Design review of the part built by this model. Coordinates are the model's own, in mm. Face numbers are marked on the shaded views. A direction names the side the tool comes from. Round coordinates to 2 decimals unless told otherwise and drop trailing zeros. Loops run counter-clockwise (first coordinate to the right, second up) from the corner with the lowest first, then second, coordinate; pieces in that order, holes last. Notation, with made-up numbers: M -14.75,82 L 41.25,82 A31 ccw 41.25,108 Z; hole C -39,8 d6. An arc over 180 degrees is marked long. Answer as CSV lines item,"result". Start each with the question number.
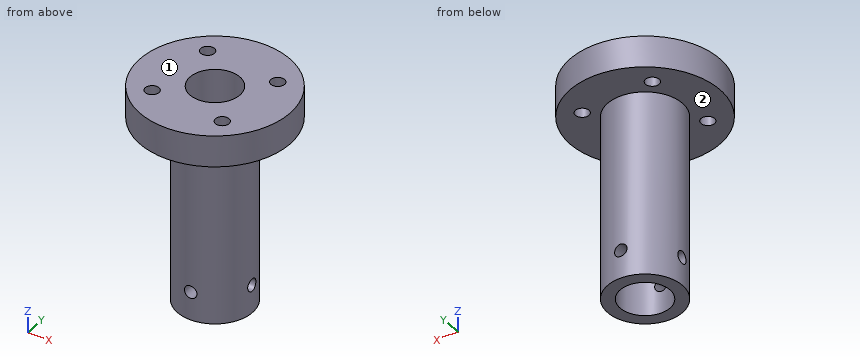
from build123d import *

# Parameters (mm, degrees)
SKIZZE1_R                            = 12.5
AUFSATZ_LINEAR_AUSTRAGEN1_DEPTH      = 40
SCHNITT_LINEAR_START                 = 30
SKIZZE4_R                            = 15
SKIZZE4_R_2                          = 12
SCHNITT_LINEAR_AUSTRAGEN1_DEPTH      = 20
SKIZZE5_R                            = 1.1
SCHNITT_LINEAR_AUSTRAGEN2_DEPTH      = 20
SKIZZE6_R                            = 1
SCHNITT_LINEAR_AUSTRAGEN3_DEPTH      = 10
SKIZZE8_W                            = 5.5
SKIZZE8_H                            = 25
SCHNITT_LINEAR_AUSTRAGEN5_DEPTH      = 13.5
SCHNITT_LINEAR_AUSTRAGEN5_DEPTH_BACK = 13.5
SKIZZE9_R                            = 1
SCHNITT_LINEAR_AUSTRAGEN6_DEPTH      = 13
SCHNITT_LINEAR_AUSTRAGEN6_DEPTH_BACK = 13
SKIZZE11_R                           = 1
SCHNITT_LINEAR_AUSTRAGEN7_DEPTH      = 13
SCHNITT_LINEAR_AUSTRAGEN7_DEPTH_BACK = 13


with BuildPart() as part:
    # Skizze1 → Aufsatz-Linear austragen1 (new body)
    with BuildSketch(Plane.XY):
        Circle(SKIZZE1_R)
    extrude(amount=AUFSATZ_LINEAR_AUSTRAGEN1_DEPTH)

    # Skizze2 → Schnitt-Rotation3 (revolve, cut)
    with BuildSketch(Plane(origin=(0, 0, 0), x_dir=(0, 0, -1), z_dir=(1, 0, 0))):
        Polygon((-35, -12.5), (-35, -6), (-5, -6), (-5, -12.5), (-33.974333956, -17.5), align=None)
    revolve(axis=Axis((0, 0, 40), (0, 0, -1)), mode=Mode.SUBTRACT)

    # Skizze4 → Schnitt-Linear austragen1 (cut)
    with BuildSketch(Plane.XY.offset(SCHNITT_LINEAR_START)):
        Circle(SKIZZE4_R)
        Circle(SKIZZE4_R_2, mode=Mode.SUBTRACT)
    extrude(amount=SCHNITT_LINEAR_AUSTRAGEN1_DEPTH, mode=Mode.SUBTRACT)

    # Skizze5 → Schnitt-Linear austragen2 (cut)
    with BuildSketch(Plane.XY.offset(40)):
        with Locations((-5.457266806, 6.503717322)):
            Circle(SKIZZE5_R)
        with Locations((6.503717322, 5.457266806)):
            Circle(SKIZZE5_R)
        with Locations((5.457266806, -6.503717322)):
            Circle(SKIZZE5_R)
        with Locations((-6.503717322, -5.457266806)):
            Circle(SKIZZE5_R)
    extrude(amount=-SCHNITT_LINEAR_AUSTRAGEN2_DEPTH, mode=Mode.SUBTRACT)

    # Skizze6 → Schnitt-Linear austragen3 (cut)
    with BuildSketch(Plane(origin=(0, 0, 0), x_dir=(-1, 0, 0), z_dir=(0, 0, -1))):
        with Locations((-2.25, 0)):
            Circle(SKIZZE6_R)
        with Locations((0, 2.25)):
            Circle(SKIZZE6_R)
        with Locations((2.25, 0)):
            Circle(SKIZZE6_R)
        with Locations((0, -2.25)):
            Circle(SKIZZE6_R)
    extrude(amount=-SCHNITT_LINEAR_AUSTRAGEN3_DEPTH, mode=Mode.SUBTRACT)

    # Skizze7 → Schnitt-Rotation4 (revolve, cut)
    with BuildSketch(Plane(origin=(0, 0, 0), x_dir=(0, 0, -1), z_dir=(1, 0, 0))):
        Polygon((-5.069914244, 0), (-35.074978214, 0), (-40, 0), (-42.313201415, 0), (-42.313201415, -4), (-40, -4), (-35, -4), (-5, -4), align=None)
    revolve(axis=Axis((0, 0, 40), (0, 0, -1)), mode=Mode.SUBTRACT)

    # Skizze8 → Schnitt-Linear austragen5 (cut, two sides)
    with BuildSketch(Plane(origin=(0, 0, 0), x_dir=(0, 0, -1), z_dir=(1, 0, 0))) as schnitt_linear_austragen5_sk:
        with Locations((-2.75, 0)):
            Rectangle(SKIZZE8_W, SKIZZE8_H)
    extrude(amount=SCHNITT_LINEAR_AUSTRAGEN5_DEPTH, mode=Mode.SUBTRACT)
    extrude(schnitt_linear_austragen5_sk.sketch, amount=-SCHNITT_LINEAR_AUSTRAGEN5_DEPTH_BACK, mode=Mode.SUBTRACT)

    # Skizze9 → Schnitt-Linear austragen6 (cut, two sides)
    with BuildSketch(Plane(origin=(0, 0, 0), x_dir=(0, 0, -1), z_dir=(1, 0, 0))) as schnitt_linear_austragen6_sk:
        with Locations((-10, 0)):
            Circle(SKIZZE9_R)
    extrude(amount=SCHNITT_LINEAR_AUSTRAGEN6_DEPTH, mode=Mode.SUBTRACT)
    extrude(schnitt_linear_austragen6_sk.sketch, amount=-SCHNITT_LINEAR_AUSTRAGEN6_DEPTH_BACK, mode=Mode.SUBTRACT)

    # Skizze11 → Schnitt-Linear austragen7 (cut, two sides)
    with BuildSketch(Plane(origin=(0, 0, 0), x_dir=(1, 0, 0), z_dir=(0, 1, 0))) as schnitt_linear_austragen7_sk:
        with Locations((0, -10)):
            Circle(SKIZZE11_R)
    extrude(amount=SCHNITT_LINEAR_AUSTRAGEN7_DEPTH, mode=Mode.SUBTRACT)
    extrude(schnitt_linear_austragen7_sk.sketch, amount=-SCHNITT_LINEAR_AUSTRAGEN7_DEPTH_BACK, mode=Mode.SUBTRACT)


solid = part.part
Item 1: Consider section C-C, the plane z = 28.5. Write out the cut boundary in (x, y).
Item 2: To check wall thickness, follow line 1 (Z direction, x = 7, y = 0.25); line 2 (Z direction, x = 0, y = 4.7); line 3 (Y direction, x = -0.75, z = 11.5). State the ranges of each line that lie inside material, in increasing order.
Item 3: Insertion check: pin 1 Ø6 at (y, z) = (-6.5, 35.5) entering from -X; pin 2 Ø3.5 at (x, y) = (-5.46, 6.5) entering from +Z; pin 3 Ø3 at (x, z) = (0, 10) entering from +Y; pin 4 Ø1 at (x, z) = (4.5, 28) entering from +Y. Each pin has a flat end and moves straight along its axis. Give the tip position at first contact, or say it passes through.
Item 4: Consider section A-A, the plane y = 0. Write out the cut boundary in (x, z).
Item 5: Consider section D-D, the plane x = 7. Write out the cut boundary in (y, z), then the cut area to 3 significant figures.
Item 6: Tool access review of the marked faces 1 and 2: name each direction out of +Z, -Z, +X, -X, +Y, -Y from which nothing blocks a thin tool from reaching the whole face with its end or side.
Found:
1,outline,"C 0,0 d12; hole C 0,0 d8"
2,line 1,"z = 35 to 40"
2,line 2,"z = 5.5 to 9, 11 to 40"
2,line 3,"y = -5.95 to -3.93, 3.93 to 5.95"
3,pin 1,"stops at x = -11.48"
3,pin 2,"stops at z = 40"
3,pin 3,"stops at y = 6"
3,pin 4,"stops at y = 4.47"
4,outline,"M -12,35 L -6,35 L -6,11 L -4,11 L -4,40 L -12,40 Z; M -6,5.5 L -4,5.5 L -4,9 L -6,9 Z; M 4,5.5 L 6,5.5 L 6,9 L 4,9 Z; M 4,11 L 6,11 L 6,35 L 12,35 L 12,40 L 4,40 Z"
5,outline,"M -9.75,35 L 4.48,35 L 4.48,40 L -9.75,40 Z; M 6.44,35 L 9.75,35 L 9.75,40 L 6.44,40 Z"
5,area,"87.7 mm^2"
6,face 1,"+Z, +X, -X, +Y, -Y"
6,face 2,"-Z"
